Geometry check sheet. Reference: the model listing, model coordinates, mm. Round coordinates to 2 decimals unless told otherwise and drop trailing zeros. Order: outer loops, then holes, each group sorted by start corner. A loop starts at its lowest first (then second) coordinate and runs counter-clockwise, first axis right, second up. Notation, with made-up numbers: (74.25, 77.25) - (130.25, 77.25) arc R19 ccw to (130.25, 100.25) - close; hole circle Ø2 at (25, 18.25). An arc over 180 degrees is marked (long way). Write each question's results on one line, items separated by ' | '.
```python
from build123d import *

# Parameters (mm, degrees)
F0_W        = 38.1
F0_H        = 38.1
F0_W_2      = 25.4
F0_H_2      = 25.4
F1_DEPTH    = 952.5
F2_R        = 9.525
F3_DEPTH    = 76.2
F4_W        = 127
F4_H        = 25.4
F5_DEPTH    = 25.4
F6_T1_DEPTH = 133.35
F6_T3_DEPTH = 101.6
F6_T5_DEPTH = 101.6


# Not quite as in the source:
# - a fillet or chamfer that OpenCascade refuses, or shapes differently, is made with other operations: its cross-section is extruded or revolved along the edge and cut away or added


with BuildPart() as f1:
    # F0 (on Front) → F1 (new body, symmetric)
    with BuildSketch(Plane.XZ):
        Rectangle(F0_W, F0_H)
        Rectangle(F0_W_2, F0_H_2, mode=Mode.SUBTRACT)
    extrude(amount=F1_DEPTH, both=True)

    # F2 (on face) → F3 (cut)
    with BuildSketch(Plane.XY.offset(19.05)):
        with Locations((0, -889)):
            Circle(F2_R)
        with Locations((0, 889)):
            Circle(F2_R)
    extrude(amount=-F3_DEPTH, mode=Mode.SUBTRACT)

    # F4 (on Right) → F5 (cut)
    with BuildSketch(Plane.YZ):
        with Locations((901.7, 0)):
            Rectangle(F4_W, F4_H)
        with Locations((-901.7, 0)):
            Rectangle(F4_W, F4_H)
    extrude(amount=-F5_DEPTH, mode=Mode.SUBTRACT)

    # F6: fillet of radius 19.05 on 6 edges, made by hand

    # F6_s2 → F6_t1 (cut)
    with BuildSketch(Plane.XY.offset(-66.675)):
        with BuildLine():
            ThreePointArc((19.05, -933.45), (13.4703841816, -946.9203841816), (0, -952.5))
            Line((0, -952.5), (19.05, -952.5))
            Line((19.05, -952.5), (19.05, -933.45))
        make_face()
        with BuildLine():
            ThreePointArc((19.05, 933.45), (13.4703841816, 946.9203841816), (0, 952.5))
            Line((0, 952.5), (19.05, 952.5))
            Line((19.05, 952.5), (19.05, 933.45))
        make_face()
    extrude(amount=F6_T1_DEPTH, mode=Mode.SUBTRACT)

    # F6_s4 → F6_t3 (cut)
    with BuildSketch(Plane.XY.offset(-34.925)):
        with BuildLine():
            ThreePointArc((-19.05, -933.45), (-13.4703841816, -946.9203841816), (0, -952.5))
            Line((0, -952.5), (-19.05, -952.5))
            Line((-19.05, -952.5), (-19.05, -933.45))
        make_face()
        with BuildLine():
            ThreePointArc((-19.05, 933.45), (-13.4703841816, 946.9203841816), (0, 952.5))
            Line((0, 952.5), (-19.05, 952.5))
            Line((-19.05, 952.5), (-19.05, 933.45))
        make_face()
    extrude(amount=F6_T3_DEPTH, mode=Mode.SUBTRACT)

    # F6_s6 → F6_t5 (cut)
    with BuildSketch(Plane.XY.offset(-66.675)):
        with BuildLine():
            ThreePointArc((-19.05, -933.45), (-13.4703841816, -946.9203841816), (0, -952.5))
            Line((0, -952.5), (-19.05, -952.5))
            Line((-19.05, -952.5), (-19.05, -933.45))
        make_face()
        with BuildLine():
            ThreePointArc((-19.05, 933.45), (-13.4703841816, 946.9203841816), (0, 952.5))
            Line((0, 952.5), (-19.05, 952.5))
            Line((-19.05, 952.5), (-19.05, 933.45))
        make_face()
    extrude(amount=F6_T5_DEPTH, mode=Mode.SUBTRACT)


solid = f1.part
```
(1) Material ranges on line 1 (X direction, y = -193, z = 8.5); line 2 (X direction, y = -889, z = 16) (3 decimals), recorded low to high.
Answers follow:
line 1: -19.05 to -12.7, 12.7 to 19.05 | line 2: -19.05 to -9.525, 9.525 to 19.05
(2) Section check B-B (y = -749). Record the cut outline in (x, z).
Answers follow:
outline: (-19.05, -19.05) - (19.05, -19.05) - (19.05, 19.05) - (-19.05, 19.05) - close; hole (-12.7, -12.7) - (12.7, -12.7) - (12.7, 12.7) - (-12.7, 12.7) - close
(3) Draft check along X on faces 1 (the face through (1, -13, -12.7)), 2 (the face through (1, -13, 12.7)), 3 (the face through (19.05, -13, 0)), 4 (the face through (0, -13, 19.05)). Enter one of: released by +X, released by -X, zero draft, split by the parting line, or undercut.
Answers follow:
face 1: undercut | face 2: undercut | face 3: released by +X | face 4: zero draft
(4) Depth check by flat-ended pin: pin 1 Ø10 at (x, z) = (-3, 5.5) entering from -Y; pin 2 Ø1.9 at (x, z) = (-15.5, -6) entering from -Y; pin 3 Ø12 at (x, z) = (-7.5, -14) entering from -Y; pin 4 Ø5 at (x, z) = (-16, 0.5) entering from +Y. Enter the tip coordinate at first touch or a pass-through.
Answers follow:
pin 1: through | pin 2: y = -838.2 | pin 3: y = -952.44 | pin 4: y = 838.2
(5) Section check A-A (z = 2). Record the cut outline in (x, y).
Answers follow:
outline: (-19.05, -838.2) - (-12.7, -838.2) - (-12.7, 838.2) - (-19.05, 838.2) - close; (12.7, -947.65) arc R19.05 ccw to (19.05, -933.45) - (19.05, 933.45) arc R19.05 ccw to (12.7, 947.65) - close
